```python
from build123d import *

# Parameters (mm, degrees)
BOSS_EXTRUDE1_DEPTH = 35
FILLET9_R           = 30
FILLET12_R          = 30
SHELL2_T            = -2


with BuildPart() as part:
    # Sketch1 → Boss-Extrude1 (new body)
    with BuildSketch(Plane(origin=(0, 0, 0), x_dir=(1, 0, 0), z_dir=(0, 1, 0))):
        Polygon((100, 41.421356237), (41.421356237, 100), (-41.421356237, 100), (-100, 41.421356237), (-100, -41.421356237), (-41.421356237, -100), (41.421356237, -100), (100, -41.421356237), align=None)
    extrude(amount=BOSS_EXTRUDE1_DEPTH)

    # Fillet9
    fillet9_edges = [part.edges().sort_by_distance(p)[0] for p in [
        (41.421356237, 17.5, -100),
        (100, 17.5, -41.421356237),
        (100, 17.5, 41.421356237),
        (41.421356237, 17.5, 100),
        (-41.421356237, 17.5, 100),
        (-100, 17.5, 41.421356237),
        (-100, 17.5, -41.421356237),
        (-41.421356237, 17.5, -100),
    ]]
    fillet(fillet9_edges, radius=FILLET9_R)

    # Fillet12
    fillet12_edges = [part.edges().sort_by_distance(p)[0] for p in [
        (-70.710678119, 35, 70.710678119),
        (-100, 35, 0),
        (0, 35, -100),
        (-70.710678119, 35, -70.710678119),
        (0, 35, 100),
        (70.710678119, 35, 70.710678119),
        (100, 35, 0),
        (70.710678119, 35, -70.710678119),
        (-40.475452337, 35, 97.716385975),
        (40.475452337, 35, 97.716385975),
        (97.716385975, 35, 40.475452337),
        (97.716385975, 35, -40.475452337),
        (40.475452337, 35, -97.716385975),
        (-40.475452337, 35, -97.716385975),
        (-97.716385975, 35, -40.475452337),
        (-97.716385975, 35, 40.475452337),
    ]]
    fillet(fillet12_edges, radius=FILLET12_R)

    # Shell2
    shell2_openings = [part.faces().sort_by_distance(p)[0] for p in [
        (0, 0, 0),
    ]]
    offset(amount=SHELL2_T, openings=shell2_openings, kind=Kind.INTERSECTION)


solid = part.part
```
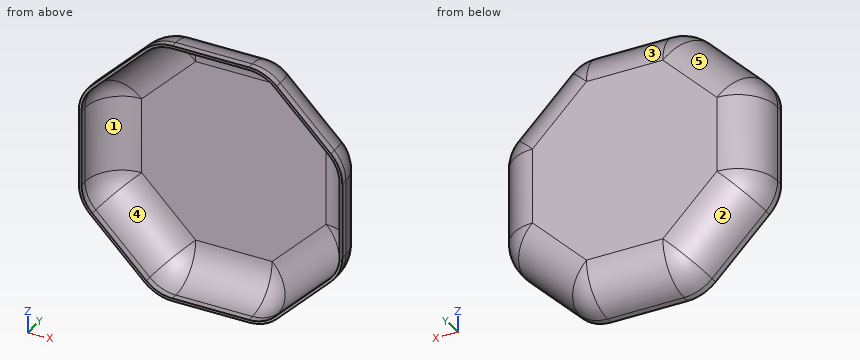
Here's how the part is built. I have some questions about the finished solid (model axes, mm). Face numbers are marked on the shaded views. A direction names the side the tool comes from. Round coordinates to 2 decimals unless told otherwise and drop trailing zeros. Write each loop counter-clockwise with the first axis right and the second up, starting at its lowest first coordinate (ties: lowest second). Pieces come first, ordered by that corner, then holes. Notation, with made-up numbers: M -4,-36 L 17,-36 A16 ccw 17,-12 Z; hole C 62.25,1.25 d1. An arc over 180 degrees is marked long. Answer as CSV lines item,"result". Start each with the question number.
1. On a 3-axis mill with a long thin cutter (end or side, diameter ignored), from which of +Z, -Z, +X, -X, +Y, -Y can I reach the whole of each face in a straight line? I mean the marked faces 1 and 2. Say none if no direction works.
2. Suppose I cut it at B-B on z = -26. Write out the boundary of the cut face in (x, y).
3. I need wall thicknesses on probe 1 along X at (y, z) = (2.5, -7.5); probe 2 along Y at (x, z) = (-47.5, -43); probe 3 along X at (y, z) = (29, 56). Which ranges of each line are inside material? Lowest first, please.
4. Thinking about a two-plate mould opening in X: for the marked faces 3, 4 and 5, which applies, released by +X, released by -X, zero draft, split by the parting line, or undercut?
5. I'm going to push flat-ended pins straight in: pin 1 Ø1.5 at (x, z) = (66, -60.5) entering from +Y; pin 2 Ø2 at (y, z) = (6, 43) entering from -X; pin 3 Ø10 at (y, z) = (11, 36.5) entering from +X. Where does each tip first touch, or does it pass through?
Check result:
1,face 1,"-Y"
1,face 2,"-Z, -X, +Y"
2,outline,"M -100,0 L -98,0 L -98,5 A28 cw -70,33 L 70,33 A28 cw 98,5 L 98,0 L 100,0 L 100,5 A30 ccw 70,35 L -70,35 A30 ccw -100,5 Z"
3,probe 1,"x = -100 to -98, 98 to 100"
3,probe 2,"y = 33 to 35"
3,probe 3,"x = -68.45 to -63.39, 63.39 to 68.45"
4,face 3,"zero draft"
4,face 4,"undercut"
4,face 5,"released by -X"
5,pin 1,"stops at y = 28.46"
5,pin 2,"stops at x = -97.02"
5,pin 3,"stops at x = 99.64"
